from build123d import *

# Parameters (mm, degrees)
SKETCH2_R           = 38
SKETCH2_R_2         = 25
BOSS_EXTRUDE2_DEPTH = 9.5
SKETCH1_R           = 3
CUT_EXTRUDE1_DEPTH  = 9.5
CIRPATTERN1_COUNT   = 3


with BuildPart() as part:
    # Sketch2 → Boss-Extrude2 (new body)
    with BuildSketch(Plane.XY):
        Circle(SKETCH2_R)
        Circle(SKETCH2_R_2, mode=Mode.SUBTRACT)
    extrude(amount=BOSS_EXTRUDE2_DEPTH)

    # Sketch1 → Cut-Extrude1 (cut)
    with BuildSketch(Plane.XY):
        with Locations((0, 30)):
            Circle(SKETCH1_R)
        with BuildLine():
            ThreePointArc((-0.208321274, 32.992758301), (2.046342613, 32.193736974), (3, 30))
            ThreePointArc((3, 30), (2.121320344, 27.878679656), (0, 27))
            ThreePointArc((0, 27), (22.353121455, 17.28106259), (30.490756455, -5.694983191))
            ThreePointArc((30.490756455, -5.694983191), (33.588054611, -2.905861808), (36.483463602, -5.904038041))
            ThreePointArc((36.483463602, -5.904038041), (36.476196349, -6.112726104), (36.454429797, -6.320403108))
            ThreePointArc((36.454429797, -6.320403108), (27.494508002, 22.075827712), (-0.208321274, 32.992758301))
        make_face()
        with Locations((33.483463602, -5.904038041)):
            Circle(SKETCH1_R)
    cut_extrude1 = extrude(amount=CUT_EXTRUDE1_DEPTH, mode=Mode.SUBTRACT)

    # CirPattern1: Cut-Extrude1 ×3 about axis
    cirpattern1_axis = Axis((0, 0, 0), (0, 0, 1))
    for i in range(1, CIRPATTERN1_COUNT):
        add(cut_extrude1.rotate(cirpattern1_axis, i * 360 / CIRPATTERN1_COUNT), mode=Mode.SUBTRACT)


solid = part.part
The listing builds one solid part. Answer for the finished solid, in the listing's coordinates (mm). A direction names the side the tool comes from. Coordinates: 2 decimals unless noted, no trailing zeros. Order: outer loops, then holes, each group sorted by start corner. A loop starts at its lowest first (then second) coordinate and runs counter-clockwise, first axis right, second up.
Q1. A cutting plane is placed at C-C, the plane x = 17. Write down the section's boundary in (y, z), and give its area (3 significant figures).
Q2. Which of the six approach directions +Z, -Z, +X, -X, +Y, -Y give full straight-line access (tool end or side, diameter ignored) to faces 1 (the face through (-23, -11, 0)), 2 (the face through (-3, 30, 5))?
Q3. A cutting plane is placed at D-D, the plane z = 6.5. Write down the section's boundary in (x, y).
Q4. A cutting plane is placed at A-A, the plane y = -31. Write down the section's boundary in (x, z).
Q5. Given P1, Ø12, axis at x = 3, y = -17, coming from the -Z side; P2, Ø1, axis at x = 28, z = 6.5, coming from the -Y side (3 decimals), each flat-ended and moving along its own axis, determine where each tip first touches the part or whether it passes through.
Q6. Consider line 1 (Y direction, x = 3, z = 3.5); line 2 (Y direction, x = 0, z = 7); line 3 (X direction, y = 22, z = 8.25). Determine where each line is inside the solid, lowest interval first.
Q7. A cutting plane is placed at B-B, the plane y = 3. Write down the section's boundary in (x, z).
Q8. For a pull along Y with two mould halves and no side action, classify faces 3 (the face through (-23, -11, 9.5)), 4 (the face through (-32.74, 13.18, 4.68)), 5 (the face through (17.535, -33.713, 4.684)) as pulls with the +Y half, pulls with the -Y half, needs draft (parallel to the pull), parting line crosses it, or undercut.
Answers follow:
1. outline: (-33.99, 0) - (-29.78, 0) - (-29.78, 9.5) - (-33.99, 9.5) - close; (-21.25, 0) - (-18.33, 0) - (-18.33, 9.5) - (-21.25, 9.5) - close; (18.33, 0) - (21.84, 0) - (21.84, 9.5) - (18.33, 9.5) - close; (29.75, 0) - (33.99, 0) - (33.99, 9.5) - (29.75, 9.5) - close
1. area: 141 mm2
2. face 1: -Z, +X, -X, +Y, -Y
2. face 2: +Z, -Z
3. outline: circle Ø76 at (0, 0); hole (-28.47, -16.68) arc R3 ccw to (-23.38, -13.5) arc R30.57 cw to (-10.31, 29.25) arc R3 ccw to (-12.75, 34.73) arc R34.6 ccw to start; hole circle Ø50 at (0, 0); hole (-23.7, -28.41) arc R34.6 ccw to (28.68, -16.32) arc R3 ccw to (23.38, -13.5) arc R30.57 cw to (-20.18, -23.56) arc R3 ccw to start; hole (-0.21, 32.99) arc R3 ccw to (0, 27) arc R30.57 cw to (30.49, -5.69) arc R3 ccw to (36.45, -6.32) arc R34.6 ccw to start
4. outline: (-21.98, 0) - (-19.88, 0) - (-19.88, 9.5) - (-21.98, 9.5) - close; (15.06, 0) - (21.98, 0) - (21.98, 9.5) - (15.06, 9.5) - close
5. P1: passes through
5. P2: stops at y = -26.225
6. line 1: y = -37.88 to -35.31, -28.17 to -24.82, 24.82 to 26.85, 33.07 to 37.88
6. line 2: y = -38 to -35.65, -28.63 to -25, 25 to 27, 33.01 to 38
6. line 3: x = -30.98 to -28.47, -19.84 to -11.87, 11.87 to 16.75, 27.57 to 30.98
7. outline: (-37.88, 0) - (-34.38, 0) - (-34.38, 9.5) - (-37.88, 9.5) - close; (-27.45, 0) - (-24.82, 0) - (-24.82, 9.5) - (-27.45, 9.5) - close; (24.82, 0) - (29.85, 0) - (29.85, 9.5) - (24.82, 9.5) - close; (36.49, 0) - (37.88, 0) - (37.88, 9.5) - (36.49, 9.5) - close
8. face 3: needs draft
8. face 4: undercut
8. face 5: parting line crosses it
